from build123d import *

# Parameters (mm, degrees)
SKETCH1_W           = 457.2
SKETCH1_H           = 1244.6
BOSS_EXTRUDE1_DEPTH = 63.5
SKETCH4_W           = 457.2
SKETCH4_H           = 63.5
BOSS_EXTRUDE2_DEPTH = 266.7
CUT_EXTRUDE7_DEPTH  = 100.076


with BuildPart() as part:
    # Sketch1 → Boss-Extrude1 (new body)
    with BuildSketch(Plane(origin=(0, 0, 0), x_dir=(1, 0, 0), z_dir=(0, 1, 0))):
        with Locations((228.6, 622.3)):
            Rectangle(SKETCH1_W, SKETCH1_H)
    extrude(amount=BOSS_EXTRUDE1_DEPTH)

    # Sketch4 → Boss-Extrude2 (add)
    with BuildSketch(Plane(origin=(0, 63.5, 0), x_dir=(1, 0, 0), z_dir=(0, 1, 0))):
        with Locations((228.6, 1212.85)):
            Rectangle(SKETCH4_W, SKETCH4_H)
    boss_extrude2 = extrude(amount=BOSS_EXTRUDE2_DEPTH)

    # Mirror7: Boss-Extrude2 across plane
    add(boss_extrude2.mirror(Plane(origin=(0, 0, -622.3), x_dir=(1, 0, 0), z_dir=(0, 0, -1))))

    # Sketch11 → Cut-Extrude7 (cut)
    with BuildSketch(Plane.XY.offset(-1181.1)):
        Polygon((0, 63.5), (0, 330.2), (457.2, 330.2), (457.2, 229.907191107), align=None)
    cut_extrude7 = extrude(amount=-CUT_EXTRUDE7_DEPTH, mode=Mode.SUBTRACT)

    # Mirror8: Cut-Extrude7 across plane
    add(cut_extrude7.mirror(Plane(origin=(0, 0, -622.3), x_dir=(1, 0, 0), z_dir=(0, 0, -1))), mode=Mode.SUBTRACT)


solid = part.part
Source: CAD feature listing. Evaluate the final solid. Frame: model axes, mm. A direction names the side the tool comes from. Give positions to 0.01 mm unless a question says otherwise; leave off trailing zeros. Write each loop counter-clockwise with the first axis right and the second up, starting at its lowest first coordinate (ties: lowest second). Pieces come first, ordered by that corner, then holes. Notation, with made-up numbers: (-24, 83) -> (18, 83) arc R28 cw to (18, 122) -> close; hole circle Ø3 at (-4, 52.5). An arc over 180 degrees is marked (long way). Write item = value, one per line.
Q1. Mould query, pull axis Z, two halves, no side actions, for faces 1 (the face through (327, 109, -63.5)), 2 (the face through (231.8, 147.87, -1212.41)), 3 (the face through (276, 88, 0)), 4 (the face through (327, 109, -1181.1)). Classes: +Z half, -Z half, draft (parallel to the pull), parting line (faces both ways), or undercut.
Here are the results:
face_1 = undercut
face_2 = draft
face_3 = +Z half
face_4 = undercut
Q2. Reachability of faces 5 (the face through (225, 63.5, -630)), 6 (the face through (457.2, 62, -769)) from +Z, -Z, +X, -X, +Y, -Y: full face, straight path, thin tool, end or side. Return the list, or none.
Here are the results:
face_5 = +X, -X, +Y
face_6 = +Z, -Z, +X, +Y, -Y
Q3. Cut plane D-D on z = -115. Return loops of the section in (x, y).
Here are the results:
outline = (0, 0) -> (457.2, 0) -> (457.2, 63.5) -> (0, 63.5) -> close
Q4. First-contact query: pin 1 (1.5 mm diameter, centred on x = 141, z = -592.5, fed in from +Y). Flat tip, straight axial feed; report the tip coordinate or a pass-through.
Here are the results:
pin_1 = 63.5
Q5. Cut plane A-A on y = 117. Return loops of the section in (x, z), then the cut area to 3 significant figures.
Here are the results:
outline = (146.99, -1244.6) -> (457.2, -1244.6) -> (457.2, -1181.1) -> (146.99, -1181.1) -> close; (146.99, -63.5) -> (457.2, -63.5) -> (457.2, 0) -> (146.99, 0) -> close
area = 39,400 mm²
Q6. Cut plane B-B on x = 292.5. Return loops of the section in (y, z), then the cut area to 3 significant figures.
Here are the results:
outline = (0, -1244.6) -> (169.96, -1244.6) -> (169.96, -1181.1) -> (63.5, -1181.1) -> (63.5, -63.5) -> (169.96, -63.5) -> (169.96, 0) -> (0, 0) -> close
area = 92,600 mm²
Q7. Line query: line 1 (Z direction, x = 352, y = 114); line 2 (Y direction, x = 64.5, z = -1088). Output: solid intervals per line, ascending. Write a range as from..to.
Here are the results:
line_1 = -1244.6..-1181.1, -63.5..0
line_2 = 0..63.5
Q8. Cut plane C-C on y = 188.5. Return loops of the section in (x, z), then the cut area to 3 significant figures.
Here are the results:
outline = (343.43, -1244.6) -> (457.2, -1244.6) -> (457.2, -1181.1) -> (343.43, -1181.1) -> close; (343.43, -63.5) -> (457.2, -63.5) -> (457.2, 0) -> (343.43, 0) -> close
area = 14,400 mm²
